Work out the finished part from the listing and answer in its coordinate system (mm). A direction names the side the tool comes from. Round coordinates to 2 decimals unless told otherwise and drop trailing zeros. Loops run counter-clockwise (first coordinate to the right, second up) from the corner with the lowest first, then second, coordinate; pieces in that order, holes last. Notation, with made-up numbers: M 30,-39 L 46,-39 A24 cw 46,-29 Z; hole C 74.5,35 d3. An arc over 180 degrees is marked long. One line per item, written item: value.
```python
from build123d import *

# Parameters (mm, degrees)
PAD_DEPTH       = 20
PAD001_DEPTH    = 20
SKETCH002_W     = 7.534247
SKETCH002_H     = 18.356169
PAD002_DEPTH    = 56
POCKET_DEPTH    = 5
POCKET001_DEPTH = 40.001
POCKET002_DEPTH = 56.692633
POCKET003_DEPTH = 74.843939


with BuildPart() as part:
    # Sketch → Pad (new body)
    with BuildSketch(Plane.XY):
        Polygon((-40, 30), (-20, 50), (10, 50), (30, 30), (38.36837, 0), (13.027784, -24.842939), (-20, -24.434219), (-39.901337, 0), align=None)
    extrude(amount=PAD_DEPTH)

    # Sketch001 (on Face10 of Pad) → Pad001 (join)
    with BuildSketch(Plane.XY.offset(20)):
        Polygon((-15.172565, 34.803986), (-27.22736, 18.502615), (-23.939688, -4.237112), (-6.268454, -12.456291), (17.019218, -7.524785), (23.183601, 16.584805), (8.800038, 36.036858), align=None)
    extrude(amount=PAD001_DEPTH)

    # Sketch002 (on Face18 of Pad001) → Pad002 (join)
    with BuildSketch(Plane.XY.offset(40)):
        with Locations((-14.5561395, 12.3382465)):
            Rectangle(SKETCH002_W, SKETCH002_H)
    extrude(amount=PAD002_DEPTH)

    # Sketch003 (on Face18 of Pad002) → Pocket (cut)
    with BuildSketch(Plane.XY.offset(40)):
        Polygon((1.600922, 18.280258), (1.261332, 3.813683), (7.577722, 6.734164), (7.781478, 14.001411), align=None)
    extrude(amount=-POCKET_DEPTH, mode=Mode.SUBTRACT)

    # Sketch004 (on Face18 of Pocket) → Pocket001 (cut, through all)
    with BuildSketch(Plane.XY.offset(40)):
        Polygon((-6.566783, 28.06591), (2.529732, 32.209877), (7.987638, 26.145536), (4.045817, 20.788698), (-3.736759, 18.565105), align=None)
    extrude(amount=-POCKET001_DEPTH, mode=Mode.SUBTRACT)

    # Sketch005 (on Face24 of Pocket001) → Pocket002 (cut, through all)
    with BuildSketch(Plane(origin=(-18.323263, 0, 0), x_dir=(0, -1, 0), z_dir=(-1, 0, 0))):
        Polygon((-16.897299, 81.534035), (-9.615451, 84.923866), (-9.615451, 61.822807), (-13.507476, 61.571709), align=None)
    extrude(amount=-POCKET002_DEPTH, mode=Mode.SUBTRACT)

    # Sketch006 (on Face3 of Pocket002) → Pocket003 (cut, through all)
    with BuildSketch(Plane(origin=(0, 50, 0), x_dir=(-1, 0, 0), z_dir=(0, 1, 0))):
        Polygon((-5.278273, 8.691591), (12.302259, 16.17749), (16.158628, 8.464747), (13.209641, 2.566766), (2.434486, 2.566766), align=None)
    extrude(amount=-POCKET003_DEPTH, mode=Mode.SUBTRACT)


solid = part.part
```
1) Each of these flat-tipped pins is pushed along its axis until it touches: pin 1 (4 mm diameter, centred on x = -14, z = 74, fed in from -Y); pin 2 (3 mm diameter, centred on x = -9, y = 28.5, fed in from +Z); pin 3 (4 mm diameter, centred on x = -13, z = 78.5, fed in from +Y); pin 4 (10 mm diameter, centred on y = 28.5, z = 52.5, fed in from -X). Where does it stop, or does it pass through?
Check values:
pin 1: y = 3.16
pin 2: z = 40
pin 3: y = 21.52
pin 4: through
2) Find section B-B (z = 67). Give the vertices of the cut face in (x, y).
Check values:
outline: M -18.32,3.16 L -10.79,3.16 L -10.79,9.62 L -18.32,9.62 Z; M -18.32,14.43 L -10.79,14.43 L -10.79,21.52 L -18.32,21.52 Z
3) Find section C-C (z = 30.5). Give the vertices of the cut face in (x, y).
Check values:
outline: M -27.23,18.5 L -23.94,-4.24 L -6.27,-12.46 L 17.02,-7.52 L 23.18,16.58 L 8.8,36.04 L -15.17,34.8 Z; hole M -6.57,28.07 L -3.74,18.57 L 4.05,20.79 L 7.99,26.15 L 2.53,32.21 Z
4) Find the intervals of material crossed by probe 1 along Z at (x, y) = (-11, -14); probe 2 along Z at (x, y) = (-24.5, -9.5); probe 3 along X at (y, z) = (9, 13), in increasing order. Write a range as from..to.
Check values:
probe 1: 0..2.57, 15.62..20
probe 2: 0..20
probe 3: -39.93..-13.89, -4.84..35.86
5) Find section A-A (y = 44). Give the vertices of the cut face in (x, z), then the cut area to 3 significant figures.
Check values:
outline: M -26,0 L 16,0 L 16,20 L -26,20 Z; hole M -16.16,8.46 L -13.21,2.57 L -2.43,2.57 L 5.28,8.69 L -12.3,16.18 Z
area: 661 mm2
6) Find section D-D (x = 20). Give the vertices of the cut face in (y, z), then the cut area to 3 significant figures.
Check values:
outline: M -18.01,0 L 40,0 L 40,20 L 20.89,20 L 20.89,40 L 4.13,40 L 4.13,20 L -18.01,20 Z
area: 1,500 mm2
7) For faces 4 (the face through (-18.323, 8, 68)), 5 (the face through (-5.132, 23.249, 1.301)), 6 (the face through (4.734, 16.111, 37.535)), 7 (the face through (-8, 13, 2.567)), determine the directions among +Z, -Z, +X, -X, +Y, -Y from which every point of the face is accessible in a straight line to the end or side of a thin tool.
Check values:
face 4: +Z, -X, +Y, -Y
face 5: +Z, -Z
face 6: +Z
face 7: +Y, -Y
8) The mould has two halves that part along Z. Classify faces 1 (the face through (-14.6, 11.5, 61.7)), 2 (the face through (-15.2, -8.3, 29.9)), 3 (the face through (0, 13, 0)): +Z half, -Z half, draft (parallel to the pull), parting line (faces both ways), or undercut.
Check values:
face 1: undercut
face 2: draft
face 3: -Z half
